Could you check a few things on this model? Use its own coordinates, in mm. A direction names the side the tool comes from. Coordinates: 2 decimals unless noted, no trailing zeros. Write each loop counter-clockwise with the first axis right and the second up, starting at its lowest first coordinate (ties: lowest second). Pieces come first, ordered by that corner, then holes.
Item 1: If I drill on probe 1 along Z at (x, y) = (245, 3.95); probe 2 along X at (y, z) = (1.5, -17); probe 3 along X at (y, z) = (5.5, -66), over which ranges is the centre line in solid material (lowest first)?
Item 2: For P1, Ø2.5, axis at x = 10, z = -10, coming from the +Y side; P2, Ø7, axis at x = 10, z = -10, coming from the -Y side; P3, Ø4, axis at x = 103.5, y = 7, coming from the -Z side, each with a flat end and sliding along its axis, tell me the tip position at first contact or that it passes through.
Item 3: Thinking about a two-plate mould opening in Z: for faces 4 (the flat face through (0, 5, -68)), 5 (the flat face through (143, 5, 0)), 6 (the flat face through (143, 5, -15)), which applies, +Z half, -Z half, draft (parallel to the pull), parting line (faces both ways), or undercut?
Item 4: Which directions (+Z, -Z, +X, -X, +Y, -Y) give clear straight access to the entire face, cutting with the end or side of a thin tool? Please do faces 1 (the flat face through (290, 5, -66)), 2 (the flat face through (280, 5, -26)), 3 (the flat face through (45, 5, -53)).
Item 5: I want a section at A-A on z = -22.5. Please give me the cut outline in (x, y), then the cut area to 3 significant figures.
Item 6: I want a section at B-B on x = 154. Please give me the cut outline in (y, z).
Item 7: I want a section at C-C on y = 3.5. Please give me the cut outline in (x, z), then the cut area to 3 significant figures.
from build123d import *

# Parameters (mm, degrees)
BOSS_EXTRU_1_DEPTH      = 10
ESQUISSE3_R             = 2
ENL_V_MAT_EXTRU_1_DEPTH = 10
CONG_1_R                = 10
ESQUISSE4_R             = 32.5
ENL_V_MAT_EXTRU_2_DEPTH = 10
ESQUISSE5_R             = 2
ENL_V_MAT_EXTRU_3_DEPTH = 10
ESQUISSE6_W             = 270
ESQUISSE6_H             = 22
ENL_V_MAT_EXTRU_4_DEPTH = 10
ESQUISSE7_R             = 2
ENL_V_MAT_EXTRU_5_DEPTH = 10
ENL_V_MAT_EXTRU_6_DEPTH = 10
ESQUISSE9_R             = 2
ENL_V_MAT_EXTRU_7_DEPTH = 10
ESQUISSE10_R            = 6
ENL_V_MAT_EXTRU_8_DEPTH = 5


with BuildPart() as part:
    # Esquisse2 → Boss.-Extru.1 (new body)
    with BuildSketch(Plane(origin=(0, 0, 0), x_dir=(1, 0, 0), z_dir=(0, 1, 0))):
        Polygon((0, 0), (290, 0), (290, 180), (275, 180), (225, 130), (65, 130), (15, 180), (0, 180), align=None)
    extrude(amount=BOSS_EXTRU_1_DEPTH)

    # Esquisse3 → Enlèv. mat.-Extru.1 (cut)
    with BuildSketch(Plane(origin=(0, 10, 0), x_dir=(1, 0, 0), z_dir=(0, 1, 0))):
        with Locations((10, 10)):
            Circle(ESQUISSE3_R)
        with Locations((280, 10)):
            Circle(ESQUISSE3_R)
    extrude(amount=-ENL_V_MAT_EXTRU_1_DEPTH, mode=Mode.SUBTRACT)

    # Congé1
    cong_1_edges = [part.edges().sort_by_distance(p)[0] for p in [
        (290, 5, 0),
        (0, 5, 0),
    ]]
    fillet(cong_1_edges, radius=CONG_1_R)

    # Esquisse4 → Enlèv. mat.-Extru.2 (cut)
    with BuildSketch(Plane.XZ):
        with Locations((239.106279441, -116.309672248)):
            Circle(ESQUISSE4_R)
        with Locations((179.153264776, -81.942630954)):
            Circle(ESQUISSE4_R)
        with Locations((110.048910395, -82.156407472)):
            Circle(ESQUISSE4_R)
        with Locations((50.309672248, -116.893720559)):
            Circle(ESQUISSE4_R)
    extrude(amount=-ENL_V_MAT_EXTRU_2_DEPTH, mode=Mode.SUBTRACT)

    # Esquisse5 → Enlèv. mat.-Extru.3 (cut)
    with BuildSketch(Plane(origin=(0, 0, 0), x_dir=(-1, 0, 0), z_dir=(0, -1, 0))):
        with Locations((-144.50570114, 101.001110603)):
            Circle(ESQUISSE5_R)
        with Locations((-199.571369329, 115.491017964)):
            Circle(ESQUISSE5_R)
        with Locations((-221.896020418, 76.419161677)):
            Circle(ESQUISSE5_R)
        with Locations((-66.897585359, 77.115673706)):
            Circle(ESQUISSE5_R)
        with Locations((-89.572479932, 115.985316824)):
            Circle(ESQUISSE5_R)
    extrude(amount=-ENL_V_MAT_EXTRU_3_DEPTH, mode=Mode.SUBTRACT)

    # Esquisse6 → Enlèv. mat.-Extru.4 (cut)
    with BuildSketch(Plane(origin=(0, 10, 0), x_dir=(1, 0, 0), z_dir=(0, 1, 0))):
        with Locations((145, 26)):
            Rectangle(ESQUISSE6_W, ESQUISSE6_H)
    extrude(amount=-ENL_V_MAT_EXTRU_4_DEPTH, mode=Mode.SUBTRACT)

    # Esquisse7 → Enlèv. mat.-Extru.5 (cut)
    with BuildSketch(Plane(origin=(0, 10, 0), x_dir=(1, 0, 0), z_dir=(0, 1, 0))):
        with Locations((10, 165)):
            Circle(ESQUISSE7_R)
        with Locations((280, 165)):
            Circle(ESQUISSE7_R)
    extrude(amount=-ENL_V_MAT_EXTRU_5_DEPTH, mode=Mode.SUBTRACT)

    # Esquisse8 → Enlèv. mat.-Extru.6 (cut)
    with BuildSketch(Plane.XZ):
        with BuildLine():
            Line((290, -124.189862343), (307.144293733, -133.59002346))
            Line((307.144293733, -133.59002346), (298.572146866, -188.47958085))
            Line((298.572146866, -188.47958085), (-31.012454314, -192.613510827))
            Line((-31.012454314, -192.613510827), (-21.06069283, -128.889942902))
            Line((-21.06069283, -128.889942902), (0, -124.189862343))
            ThreePointArc((0, -124.189862343), (145, -42), (290, -124.189862343))
        make_face()
    extrude(amount=-ENL_V_MAT_EXTRU_6_DEPTH, mode=Mode.SUBTRACT)

    # Esquisse9 → Enlèv. mat.-Extru.7 (cut)
    with BuildSketch(Plane(origin=(0, 10, 0), x_dir=(1, 0, 0), z_dir=(0, 1, 0))):
        with Locations((45, 50)):
            Circle(ESQUISSE9_R)
        with Locations((245, 50)):
            Circle(ESQUISSE9_R)
    extrude(amount=-ENL_V_MAT_EXTRU_7_DEPTH, mode=Mode.SUBTRACT)

    # Esquisse10 → Enlèv. mat.-Extru.8 (cut)
    with BuildSketch(Plane.XZ):
        with Locations((10, -10)):
            Circle(ESQUISSE10_R)
        with Locations((45, -50)):
            Circle(ESQUISSE10_R)
        with Locations((245, -50)):
            Circle(ESQUISSE10_R)
        with Locations((280, -10)):
            Circle(ESQUISSE10_R)
    extrude(amount=-ENL_V_MAT_EXTRU_8_DEPTH, mode=Mode.SUBTRACT)


solid = part.part
Response values:
1. probe 1: z = -74.76 to -56, -44 to -37, -15 to 0
1. probe 2: x = 0 to 10, 280 to 290
1. probe 3: x = 0 to 58.19, 231.81 to 290
2. P1: passes through
2. P2: stops at y = 5
2. P3: stops at z = -47.69
3. face 4: draft
3. face 5: +Z half
3. face 6: undercut
4. face 1: +Z, -Z, +X, +Y, -Y
4. face 2: +Y, -Y
4. face 3: -Y
5. outline: (0, 0) - (10, 0) - (10, 10) - (0, 10) - close; (280, 0) - (290, 0) - (290, 10) - (280, 10) - close
5. area: 200 mm2
6. outline: (0, -42.24) - (10, -42.24) - (10, -37) - (0, -37) - close; (0, -15) - (10, -15) - (10, 0) - (0, 0) - close
7. outline: (0, -124.19) arc R169 cw to (290, -124.19) - (290, -10) arc R10 ccw to (280, 0) - (10, 0) arc R10 ccw to (0, -10) - close; hole (10, -37) - (280, -37) - (280, -16) arc R6 ccw (long way) to (276.68, -15) - (13.32, -15) arc R6 ccw (long way) to (10, -16) - close; hole circle Ø12 at (45, -50); hole circle Ø12 at (245, -50)
7. area: 12,700 mm2
